Geometry check sheet. Reference: the model listing, model coordinates, mm. Face numbers are marked on the shaded views. Coordinates: 2 decimals unless noted, no trailing zeros. Order: outer loops, then holes, each group sorted by start corner. A loop starts at its lowest first (then second) coordinate and runs counter-clockwise, first axis right, second up.
```python
from build123d import *

# Parameters (mm, degrees)
SKETCH1_R           = 5.588
SKETCH1_R_2         = 5.08
BOSS_EXTRUDE1_DEPTH = 35.56
SKETCH2_R           = 5.588
SKETCH2_R_2         = 1.905
BOSS_EXTRUDE2_DEPTH = 7.62
SKETCH3_R           = 2.54
CUT_EXTRUDE1_DEPTH  = 33.02


with BuildPart() as part:
    # Sketch1 → Boss-Extrude1 (new body)
    with BuildSketch(Plane.XY):
        Circle(SKETCH1_R)
        Circle(SKETCH1_R_2, mode=Mode.SUBTRACT)
    extrude(amount=BOSS_EXTRUDE1_DEPTH)

    # Sketch2 → Boss-Extrude2 (add)
    with BuildSketch(Plane.XY.offset(35.56)):
        Circle(SKETCH2_R)
        with Locations((2.54, 0)):
            Circle(SKETCH2_R_2, mode=Mode.SUBTRACT)
    extrude(amount=BOSS_EXTRUDE2_DEPTH)

    # Sketch3 → Cut-Extrude1 (cut)
    with BuildSketch(Plane.XY.offset(43.18)):
        with Locations((-2.54, 0)):
            Circle(SKETCH3_R)
    extrude(amount=-CUT_EXTRUDE1_DEPTH, mode=Mode.SUBTRACT)


solid = part.part
```
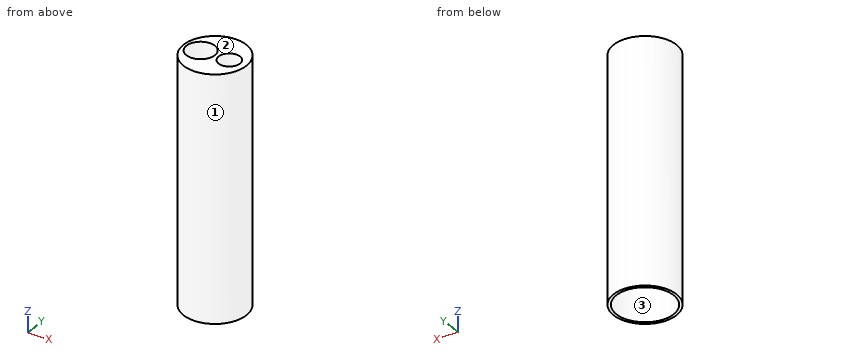
Item 1: Sectioned sample at A-A (y = 0.5). Give the number of separate pieces and of enclosed holes in the cut face, and give its area (3 significant figures).
Item 2: Sectioned sample at B-B (x = 2.54). Record the cut outline in (y, z) (3 decimals), and give its area (3 significant figures).
Item 3: Sectioned sample at C-C (z = 13). Record the cut outline in (x, y).
Item 4: Depth check by flat-ended pin: P1, Ø1, axis at x = -2, y = 2.5, coming from the -Z side; P2, Ø1, axis at x = 3.5, z = 26.5, coming from the -Y side. Enter the tip coordinate at first touch or a pass-through.
Item 5: Release check for a two-part mould opening along Y. For the marked faces 1, 2 and 3 record: pulls with the +Y half, pulls with the -Y half, needs draft (parallel to the pull), parting line crosses it, or undercut.
Item 6: Sectioned sample at D-D (y = 3.25). Record the cut outline in (x, z), and give its area (3 significant figures).
Item 7: Thickness scan on line 1 along X through (y, z) = (-1.25, 40.5); line 2 along Z through (x, y) = (0, -1.25); line 3 along Y through (x, z) = (4, 27). Record the ranges inside material, lowest first.
Geometry check:
1. separate pieces: 3
1. enclosed holes: 0
1. area: 55.1 mm2
2. outline: (-4.977, 0) - (-4.399, 0) - (-4.399, 35.56) - (-1.905, 35.56) - (-1.905, 43.18) - (-4.977, 43.18) - close; (1.905, 35.56) - (4.399, 35.56) - (4.399, 0) - (4.977, 0) - (4.977, 43.18) - (1.905, 43.18) - close
2. area: 87.9 mm2
3. outline: circle Ø11.18 at (0, 0); hole circle Ø10.16 at (0, 0)
4. P1: stops at z = 35.56
4. P2: stops at y = -4.71
5. face 1: parting line crosses it
5. face 2: needs draft
5. face 3: undercut
6. outline: (-4.55, 0) - (-3.9, 0) - (-3.9, 35.56) - (3.9, 35.56) - (3.9, 0) - (4.55, 0) - (4.55, 43.18) - (-4.55, 43.18) - close
6. area: 115 mm2
7. line 1: x = -5.45 to -4.75, -0.33 to 1.1, 3.98 to 5.45
7. line 2: z = 35.56 to 43.18
7. line 3: y = -3.9 to -3.13, 3.13 to 3.9
